Here's how the part is built. I have some questions about the finished solid (model axes, mm). Face numbers are marked on the shaded views. A direction names the side the tool comes from. Round coordinates to 2 decimals unless told otherwise and drop trailing zeros. Order: outer loops, then holes, each group sorted by start corner. A loop starts at its lowest first (then second) coordinate and runs counter-clockwise, first axis right, second up. Notation, with made-up numbers: (-36, 31) -> (6, 31) arc R10 cw to (6, 45) -> close; hole circle Ø6 at (36.25, 36). An arc over 180 degrees is marked (long way). Answer in a Markdown table with one row per item.
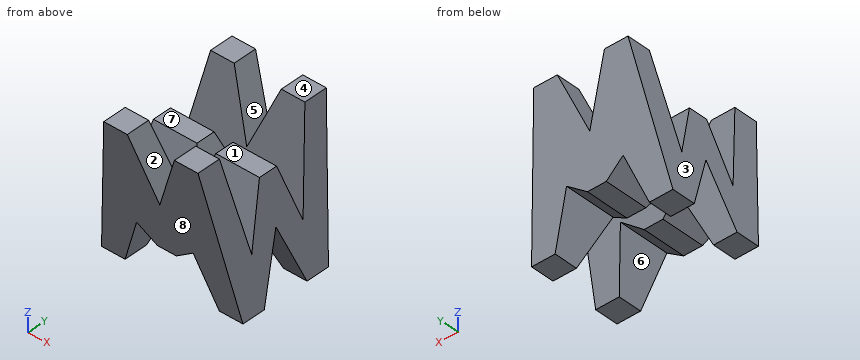
```python
from build123d import *

# Parameters (mm, degrees)
F0_W     = 38.1
F0_H     = 38.1
F1_DEPTH = 38.1
F5_DEPTH = 38.1
F7_DEPTH = 38.1


with BuildPart() as f1:
    # F0 (on Front) → F1 (new body)
    with BuildSketch(Plane.XZ):
        with Locations((19.05, 19.05)):
            Rectangle(F0_W, F0_H)
    extrude(amount=F1_DEPTH)

    # F4 (on offset) → F5 (cut)
    with BuildSketch(Plane.YZ.offset(38.1)):
        Polygon((-6.35, 38.1), (-31.75, 38.1), (-26.67, 13.394677), (-21.59, 28.575), (-16.51, 28.575), (-11.43, 13.394677), align=None)
        Polygon((-19.05, 15.875), (-25.4, 0), (-12.7, 0), align=None)
        Polygon((-31.75, 0), (-38.1, 38.1), (-38.1, 0), align=None)
        Polygon((0, 0), (0, 38.1), (-6.35, 0), align=None)
    extrude(amount=-F5_DEPTH, mode=Mode.SUBTRACT)

    # F6 (on offset) → F7 (cut)
    with BuildSketch(Plane.XZ.offset(38.1)):
        Polygon((11.43, 13.156833), (6.35, 0), (31.75, 0), (26.67, 13.156833), (21.59, 9.525), (16.51, 9.525), align=None)
        Polygon((25.4, 38.1), (12.7, 38.1), (19.05, 22.225), align=None)
        Polygon((0, 38.1), (0, 0), (6.35, 38.1), align=None)
        Polygon((31.75, 38.1), (38.1, 0), (38.1, 38.1), align=None)
    extrude(amount=-F7_DEPTH, mode=Mode.SUBTRACT)


solid = f1.part
```
1. Suppose I cut it at D-D on x = 24. Write out the boundary of the cut face in (y, z) (3 decimals), then the cut area to 3 significant figures.
Numbers:
| item | result |
|---|---|
| outline | (-37.517, 34.6) -> (-33.625, 11.248) -> (-20.901, 11.248) -> (-19.05, 15.875) -> (-17.199, 11.248) -> (-4.475, 11.248) -> (-0.583, 34.6) -> (-7.07, 34.6) -> (-11.43, 13.395) -> (-16.51, 28.575) -> (-21.59, 28.575) -> (-26.67, 13.395) -> (-31.03, 34.6) -> close |
| area | 502 mm2 |
2. Suppose I cut it at C-C on z = 7.5. Write out the boundary of the cut face in (x, y), then the cut area to 3 significant figures.
Numbers:
| item | result |
|---|---|
| outline | (1.25, -33) -> (9.25, -33) -> (9.25, -22.4) -> (1.25, -22.4) -> close; (1.25, -15.7) -> (9.25, -15.7) -> (9.25, -5.1) -> (1.25, -5.1) -> close; (28.85, -33) -> (36.85, -33) -> (36.85, -22.4) -> (28.85, -22.4) -> close; (28.85, -15.7) -> (36.85, -15.7) -> (36.85, -5.1) -> (28.85, -5.1) -> close |
| area | 339 mm2 |
3. For the marked faces 4, 5, 6, 7 and 8, which set-ups out of +Z, -Z, +X, -X, +Y, -Y let a thin tool reach every point of the face, with its end or its side?
Numbers:
| item | result |
|---|---|
| face 4 | +Z, +X, -X, +Y, -Y |
| face 5 | +Z, +Y, -Y |
| face 6 | -Z, +Y, -Y |
| face 7 | +Z, +X, -X |
| face 8 | -Z, +X, -X, -Y |
4. Suppose I cut it at B-B on z = 23. Write out the boundary of the cut face in (x, y).
Numbers:
| item | result |
|---|---|
| outline | (3.83, -35.58) -> (18.74, -35.58) -> (18.74, -28.65) -> (3.83, -28.65) -> close; (3.83, -23.46) -> (18.74, -23.46) -> (18.74, -14.64) -> (3.83, -14.64) -> close; (3.83, -9.45) -> (18.74, -9.45) -> (18.74, -2.52) -> (3.83, -2.52) -> close; (19.36, -35.58) -> (34.27, -35.58) -> (34.27, -28.65) -> (19.36, -28.65) -> close; (19.36, -23.46) -> (34.27, -23.46) -> (34.27, -14.64) -> (19.36, -14.64) -> close; (19.36, -9.45) -> (34.27, -9.45) -> (34.27, -2.52) -> (19.36, -2.52) -> close |
5. Please list where these lines run through material, in increasing order: line 1 along Y through (x, z) = (30.5, 20.5); line 2 along Y through (x, z) = (20, 17); line 3 along X through (y, z) = (-20.5, 12.5).
Numbers:
| item | result |
|---|---|
| line 1 | y = -35.17 to -28.13, -24.29 to -13.81, -9.97 to -2.93 |
| line 2 | y = -34.58 to -27.41, -25.46 to -12.64, -10.69 to -3.52 |
| line 3 | x = 2.08 to 11.18, 12.35 to 25.75, 26.92 to 36.02 |
6. We'd pull the mould along X, two halves only. Please class the marked faces 1, 2 and 3: released by +X, released by -X, zero draft, split by the parting line, or undercut.
Numbers:
| item | result |
|---|---|
| face 1 | zero draft |
| face 2 | undercut |
| face 3 | released by -X |
7. For pin 1 Ø2 at (x, z) = (14.5, 17) entering from +Y; pin 2 Ø12 at (y, z) = (-16.5, 24.5) entering from -X; pin 3 Ø1.5 at (x, y) = (19, -13) entering from -Z (3 decimals); pin 4 Ø1.5 at (y, z) = (-10, 27) entering from -X, each with a flat end and sliding along its axis, tell me the tip position at first contact or that it passes through.
Numbers:
| item | result |
|---|---|
| pin 1 | stops at y = -3.35 |
| pin 2 | stops at x = 3.08 |
| pin 3 | stops at z = 9.525 |
| pin 4 | passes through |
8. Suppose I cut it at A-A on z = 19. Write out the boundary of the cut face in (x, y), then the cut area to 3 significant figures.
Numbers:
| item | result |
|---|---|
| outline | (3.17, -34.92) -> (34.93, -34.92) -> (34.93, -27.82) -> (3.17, -27.82) -> close; (3.17, -24.79) -> (34.93, -24.79) -> (34.93, -13.31) -> (3.17, -13.31) -> close; (3.17, -10.28) -> (34.93, -10.28) -> (34.93, -3.18) -> (3.17, -3.18) -> close |
| area | 816 mm2 |
